Autodesk Inventor part; units mm, degrees
ref_plane "YZ Plane" through (0, 0, 0) normal (1, 0, 0) x (0, 1, 0)
ref_plane "XZ Plane" through (0, 0, 0) normal (0, 1, 0) x (-1, 0, 0)
ref_plane "XY Plane" through (0, 0, 0) normal (0, 0, 1) x (1, 0, 0)
sketch "スケッチ1" plane through (0, 0, 0) normal (0, 0, 1) x (1, 0, 0)
  line L0 (0, 0) -> (20, 0)
  line L1 (20, 0) -> (20, 50)
  line L2 (20, 50) -> (0, 50)
  line L3 (0, 50) -> (0, 0)
  dimension "d0" = 20
  dimension "d1" = 50
extrude "押し出し1" add sketch "スケッチ1" along normal blind 10
sketch "スケッチ2" plane through (0, 0, 10) normal (0, 0, 1) x (1, 0, 0)
  line L0 (20, 50) -> (0, 50)
  line L1 (4, 50) -> (16, 50)
  line L2 (16, 50) -> (16, 40)
  line L3 (16, 40) -> (4, 40)
  line L4 (4, 40) -> (4, 50)
  line L5 (0, 50) -> (0, 0)
  dimension "d4" = 12
  dimension "d5" = 4
  dimension "d6" = 10
extrude "押し出し2" cut sketch "スケッチ2" against normal blind 10
sketch "スケッチ3" plane through (20, 0, 0) normal (1, 0, 0) x (0, 0, -1)
  line L0 (0, 50) -> (-10, 50)
  line L1 (0, 0) -> (0, 50)
  point P0 (-5, 45)
  dimension "d9" = 5
  dimension "d10" = 5
hole "穴1" at (20, 45, 5) direction (-1, 0, 0) diameter 3 end through all
sketch "スケッチ4" plane through (0, 0, 0) normal (0, -1, 0) x (1, 0, 0)
  line L0 (0, 0) -> (0, 10)
  line L1 (0, 10) -> (20, 10)
  line L2 (0, 0) -> (20, 0)
  line L3 (20, 0) -> (20, 10)
  point P0 (5, 5)
  point P1 (15, 5)
  dimension "d18" = 5
  dimension "d19" = 5
  dimension "d20" = 5
  dimension "d21" = 5
hole "穴2" at (5, 0, 5) at (15, 0, 5) direction (0, 1, 0) diameter 2.459 depth 25 tip angle 118
sketch "スケッチ5" plane through (0, 0, 10) normal (0, 0, 1) x (1, 0, 0)
  line L0 (4, 40) -> (16, 40)
  line L1 (4, 40) -> (16, 40)
  line L2 (16, 40) -> (16, 35)
  line L3 (16, 35) -> (4, 35)
  line L4 (4, 35) -> (4, 40)
  point P0 (0, 0)
  dimension "d29" = 5
extrude "押し出し3" cut sketch "スケッチ5" against normal blind 10
properties part number "アーム支え"
Read the model definition and answer for the solid it produces. Units are mm, in the model's axes. A direction names the side the tool comes from. Coordinates: 2 decimals unless noted, no trailing zeros. Loops run counter-clockwise (first coordinate to the right, second up) from the corner with the lowest first, then second, coordinate; pieces in that order, holes last. Notation, with made-up numbers: (-32, -30.5) -> (16, -30.5) arc R12 ccw to (16, -26.5) -> close; hole circle Ø9 at (12.5, 39.5). An arc over 180 degrees is marked (long way). Return JSON: item names as keys, results as strings.
Item 1: For a pull along Y with two mould halves and no side action, classify faces 1 (the flat face through (10, 20, 0)), 2 (the cylindrical face through (17.972, 46.464, 5.325)), 3 (the flat face through (10, 35, 5)), 4 (the conical face through (5.14, 25.61, 5.16)) as +Y half, -Y half, draft (parallel to the pull), parting line (faces both ways), or undercut.
Answers:
{"face 1": "draft", "face 2": "undercut", "face 3": "+Y half", "face 4": "-Y half"}
Item 2: Find section D-D (x = 12.5). Determine the outline of the cut face in (y, z), plus the area to 3 significant figures.
Answers:
{"outline": "(0, 0) -> (35, 0) -> (35, 10) -> (0, 10) -> close", "area": "350 mm2"}
Item 3: Flat-ended cylindrical pins translate along their axes: P1, Ø2, axis at x = 5, z = 5, coming from the -Y side; P2, Ø3, axis at x = 11, z = 3, coming from the +Y side. Find the tip coordinate at first contact, or state that the pin passes through.
Answers:
{"P1": "stops at y = 25.14", "P2": "stops at y = 35"}
Item 4: For faces 5 (the flat face through (16, 43, 5)), 6 (the flat face through (2, 50, 5)), 7 (the cylindrical face through (13.78, 12.68, 5.16)), determine the directions among +Z, -Z, +X, -X, +Y, -Y from which every point of the face is accessible in a straight line to the end or side of a thin tool.
Answers:
{"face 5": "+Z, -Z, +Y", "face 6": "+Z, -Z, +X, -X, +Y", "face 7": "-Y"}
Item 5: Find the intervals of material crossed by probe 1 along X at (y, z) = (13.5, 5); probe 2 along Z at (x, y) = (18.9, 45); probe 3 along X at (y, z) = (37.5, 0.5), in increasing order.
Answers:
{"probe 1": "x = 0 to 3.77, 6.23 to 13.77, 16.23 to 20", "probe 2": "z = 0 to 3.5, 6.5 to 10", "probe 3": "x = 0 to 4, 16 to 20"}
Item 6: Find section C-C (z = 2.25). Determine the outline of the cut face in (x, y), plus the area to 3 significant figures.
Answers:
{"outline": "(0, 0) -> (20, 0) -> (20, 50) -> (16, 50) -> (16, 35) -> (4, 35) -> (4, 50) -> (0, 50) -> close", "area": "820 mm2"}
Item 7: Find section A-A (y = 45). Determine the outline of the cut face in (x, z), plus the area to 3 significant figures.
Answers:
{"outline": "(0, 0) -> (4, 0) -> (4, 3.5) -> (0, 3.5) -> close; (0, 6.5) -> (4, 6.5) -> (4, 10) -> (0, 10) -> close; (16, 0) -> (20, 0) -> (20, 3.5) -> (16, 3.5) -> close; (16, 6.5) -> (20, 6.5) -> (20, 10) -> (16, 10) -> close", "area": "56.0 mm2"}
Item 8: Find section B-B (y = 22.5). Determine the outline of the cut face in (x, z), plus the area to 3 significant figures.
Answers:
{"outline": "(0, 0) -> (20, 0) -> (20, 10) -> (0, 10) -> close; hole circle Ø2.46 at (5, 5); hole circle Ø2.46 at (15, 5)", "area": "191 mm2"}
